Part print with two shaded views. Sizes in mm from the minimum x, y, z corner. A direction names the side the tool comes from. Coordinates: 2 decimals unless noted, no trailing zeros. Write each loop counter-clockwise with the first axis right and the second up, starting at its lowest first coordinate (ties: lowest second). Pieces come first, ordered by that corner, then holes. Notation, with made-up numbers: (49.5, -25.5) - (108.5, -25.5) arc R16 cw to (108.5, 1.5) - close; hole circle Ø8 at (-19.75, 29.25). An arc over 180 degrees is marked (long way). Answer in a Markdown table with one row per item. Add a question column.
Q1. Band-saw the part on C-C (y = 4). List the corners of the cut face in (x, z) (1 decimal).
Q2. Drill centre lines: line 1 along X through (y, z) = (2.25, 5.25) (1 decimal); line 2 along Y through (x, z) = (39, 16.75) (1 decimal); line 3 along X through (y, z) = (6.5, 5.75) (1 decimal). Where is each one in solid material? Low to high. Write a range as from..to.
Q3. 3-axis set-ups, long thin cutter, end or side, ignore diameter. For the marked faces 1, 2 and 3: which of +Z, -Z, +X, -X, +Y, -Y reach the whole face in a straight line?
Q4. Band-saw the part on B-B (x = 55). List the corners of the cut face in (y, z) (1 decimal).
Q5. Pin check, flat tips, straight feed: pin 1 (3.5 mm diameter, centred on x = 66.675, z = 3.175, fed in from -Y); pin 2 (2.5 mm diameter, centred on x = 9.525, z = 22.225, fed in from +Y) (1 decimal); pin 3 (1.8 mm diameter, centred on x = 2.5, y = 4, fed in from +Z); pin 4 (2.5 mm diameter, centred on y = 4.5, z = 10, fed in from +X). Stop position of each tip, or through.
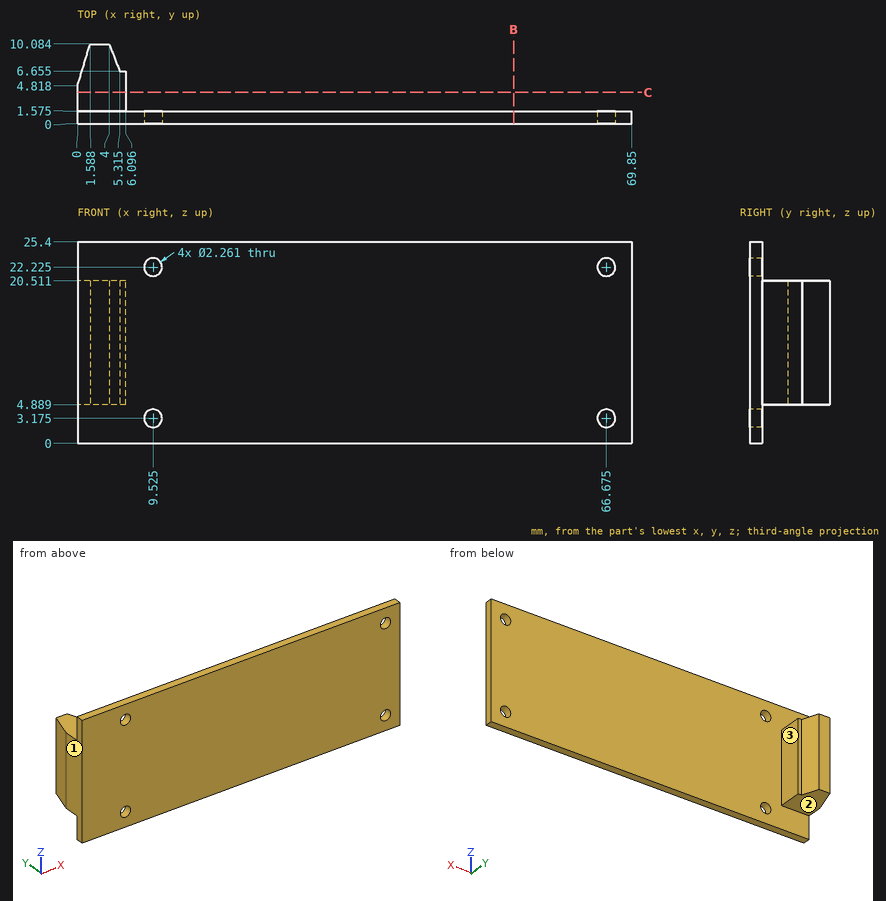
Checked values:
| question | item | result |
|---|---|---|
| 1 | outline | (0, 4.9) - (6.1, 4.9) - (6.1, 20.5) - (0, 20.5) - close |
| 2 | line 1 | x = 0..6.1 |
| 2 | line 2 | y = 0..1.6 |
| 2 | line 3 | x = 0.5..6.1 |
| 3 | face 1 | +Z, -Z, -X, +Y, -Y |
| 3 | face 2 | -Z, +X, -X, +Y |
| 3 | face 3 | +Z, -Z, +X, +Y |
| 4 | outline | (0, 0) - (1.6, 0) - (1.6, 25.4) - (0, 25.4) - close |
| 5 | pin 1 | stops at y = 0 |
| 5 | pin 2 | stops at y = 1.6 |
| 5 | pin 3 | stops at z = 20.51 |
| 5 | pin 4 | stops at x = 6.1 |
